```python
from build123d import *

# Parameters (mm, degrees)
CROQUIS1_W              = 180
CROQUIS1_H              = 60
SALIENTE_EXTRUIR1_DEPTH = 1.2
CROQUIS2_W              = 20
CROQUIS2_H              = 1.2
CROQUIS2_W_2            = 13
CROQUIS2_H_2            = 20
CROQUIS2_W_3            = 10.6
CROQUIS2_H_3            = 17.6
SALIENTE_EXTRUIR2_DEPTH = 23
REDONDEO1_R             = 8


with BuildPart() as part:
    # Croquis1 → Saliente-Extruir1 (new body)
    with BuildSketch(Plane.XY):
        with Locations((-124.847250917, 17.903225806)):
            Rectangle(CROQUIS1_W, CROQUIS1_H)
    extrude(amount=SALIENTE_EXTRUIR1_DEPTH)

    # Croquis2 → Saliente-Extruir2 (add)
    # profile 1 of 4: a face of its own
    with BuildSketch(Plane.XY.offset(1.2)):
        with Locations((-204.847250917, -11.496774194)):
            Rectangle(CROQUIS2_W, CROQUIS2_H)
    # profile 2 of 4: a face of its own
    with BuildSketch(Plane.XY.offset(1.2)):
        with Locations((-220.147250917, 37.903225806)):
            Rectangle(CROQUIS2_W_2, CROQUIS2_H_2)
        with Locations((-220.147250917, 37.903225806)):
            Rectangle(CROQUIS2_W_3, CROQUIS2_H_3, mode=Mode.SUBTRACT)
    # profile 3 of 4: a face of its own
    with BuildSketch(Plane.XY.offset(1.2)):
        with Locations((-29.547250917, 37.903225806)):
            Rectangle(CROQUIS2_W_2, CROQUIS2_H_2)
        with Locations((-29.547250917, 37.903225806)):
            Rectangle(CROQUIS2_W_3, CROQUIS2_H_3, mode=Mode.SUBTRACT)
    # profile 4 of 4: a face of its own
    with BuildSketch(Plane.XY.offset(1.2)):
        with Locations((-44.847250917, -11.496774194)):
            Rectangle(CROQUIS2_W, CROQUIS2_H)
    extrude(amount=-SALIENTE_EXTRUIR2_DEPTH)

    # Redondeo1
    redondeo1_edges = [part.edges().sort_by_distance(p)[0] for p in [
        (-34.847250917, -12.096774194, -10.3),
        (-214.847250917, -12.096774194, -10.3),
    ]]
    fillet(redondeo1_edges, radius=REDONDEO1_R)


solid = part.part
```
Geometry check sheet. Reference: the model listing, model coordinates, mm. A direction names the side the tool comes from. Coordinates: 2 decimals unless noted, no trailing zeros. Order: outer loops, then holes, each group sorted by start corner. A loop starts at its lowest first (then second) coordinate and runs counter-clockwise, first axis right, second up.
Q1. Tool access check on faces 1 (the face through (-220, 29.103, -10)), 2 (the face through (-36.047, 38, -11)), 3 (the face through (-226, 37, -21.8)). Record the directions out of +Z, -Z, +X, -X, +Y, -Y that give a thin tool (end or side, any length) a straight path to the whole face; none if there is none.
Reply:
face 1: +Z, -Z
face 2: -Z, +Y, -Y
face 3: -Z, +X, -X, +Y, -Y
Q2. Sectioned sample at B-B on y = 34.5. Record the cut outline in (x, z), and give its area (3 significant figures).
Reply:
outline: (-226.65, -21.8) - (-225.45, -21.8) - (-225.45, 1.2) - (-226.65, 1.2) - close; (-214.85, -21.8) - (-213.65, -21.8) - (-213.65, 0) - (-36.05, 0) - (-36.05, -21.8) - (-34.85, -21.8) - (-34.85, 1.2) - (-214.85, 1.2) - close; (-24.25, -21.8) - (-23.05, -21.8) - (-23.05, 1.2) - (-24.25, 1.2) - close
area: 324 mm2
Q3. Thickness scan on probe 1 along X at (y, z) = (36.5, -2); probe 2 along Z at (x, y) = (-159.5, -8); probe 3 along Y at (x, z) = (-51.5, -18.75). Record the ranges inside material, lowest first.
Reply:
probe 1: x = -226.65 to -225.45, -214.85 to -213.65, -36.05 to -34.85, -24.25 to -23.05
probe 2: z = 0 to 1.2
probe 3: y = -12.1 to -10.9
Q4. Sectioned sample at A-A on z = -11.25. Record the cut outline in (x, y).
Reply:
outline: (-226.65, 27.9) - (-213.65, 27.9) - (-213.65, 47.9) - (-226.65, 47.9) - close; (-211.06, -10.9) arc R8 ccw to (-206.85, -12.1) - (-194.85, -12.1) - (-194.85, -10.9) - close; (-54.85, -12.1) - (-42.85, -12.1) arc R8 ccw to (-38.63, -10.9) - (-54.85, -10.9) - close; (-36.05, 27.9) - (-23.05, 27.9) - (-23.05, 47.9) - (-36.05, 47.9) - close; hole (-225.45, 29.1) - (-214.85, 29.1) - (-214.85, 46.7) - (-225.45, 46.7) - close; hole (-34.85, 29.1) - (-24.25, 29.1) - (-24.25, 46.7) - (-34.85, 46.7) - close
Q5. Sectioned sample at D-D on x = -163.5. Record the cut outline in (y, z), and give its area (3 significant figures).
Reply:
outline: (-12.1, 0) - (47.9, 0) - (47.9, 1.2) - (-12.1, 1.2) - close
area: 72.0 mm2
Q6. Depth check by flat-ended pin: pin 1 Ø8.5 at (x, z) = (-32, -10.5) entering from -Y; pin 2 Ø5 at (x, z) = (-59.5, -4.5) entering from -Y; pin 3 Ø3 at (x, y) = (-44, 33) entering from -Z; pin 4 Ø1.3 at (y, z) = (-11.5, -13.5) entering from -X. Enter the tip coordinate at first touch or a pass-through.
Reply:
pin 1: stops at y = 27.9
pin 2: passes through
pin 3: stops at z = 0
pin 4: stops at x = -211.06
Q7. Sectioned sample at C-C on y = -2. Record the cut outline in (x, z).
Reply:
outline: (-214.85, 0) - (-34.85, 0) - (-34.85, 1.2) - (-214.85, 1.2) - close
Q8. Draft check along Y on faces 4 (the face through (-213.647, 38, -11)), 5 (the face through (-203, -10.897, -11)), 6 (the face through (-214.847, 38, -10)), 7 (the face through (-220, 46.703, -10)). Enter one of: released by +Y, released by -Y, zero draft, split by the parting line, or undercut.
Reply:
face 4: zero draft
face 5: released by +Y
face 6: undercut
face 7: undercut
